Design review of the part shown in the three views and the two pictorial views. Dimensions are in mm from the part's minimum x, y and z. A direction names the side the tool comes from. Give positions to 0.01 mm unless a question says otherwise; leave off trailing zeros. Order: outer loops, then holes, each group sorted by start corner. A loop starts at its lowest first (then second) coordinate and runs counter-clockwise, first axis right, second up. Notation, with made-up numbers: (56, 77) -> (95, 77) arc R8 ccw to (95, 81) -> close; hole circle Ø2 at (-23.75, 53). An arc over 180 degrees is marked (long way). Use one line per item in the form item = value.
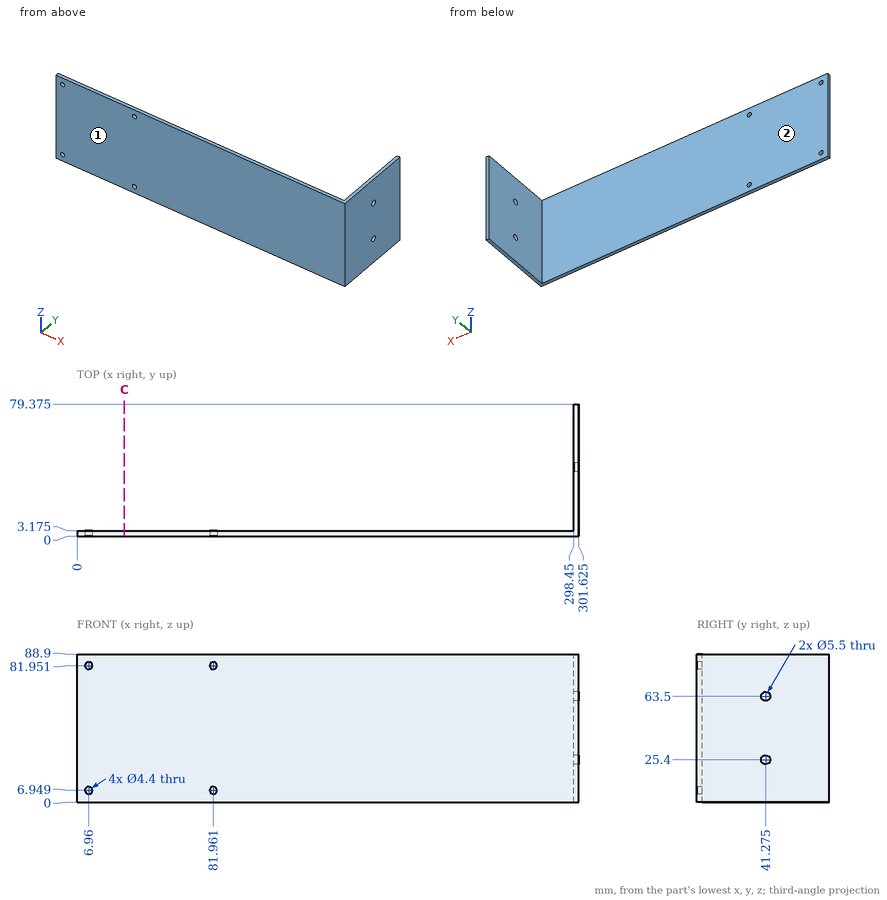
1. For L1, parallel to Y at x = 160, z = 70 (1 decimal), list the stretches that pass through material, from the lowest coordinate up.
Values:
L1 = 0 to 3.2
2. Add section C-C on x = 28.5. Give the boundary of the cut face in (y, z) (1 decimal).
Values:
outline = (0, 0) -> (3.2, 0) -> (3.2, 88.9) -> (0, 88.9) -> close
3. Tool access review of the marked faces 1 and 2: name each direction out of +Z, -Z, +X, -X, +Y, -Y from which nothing blocks a thin tool from reaching the whole face with its end or side.
Values:
face_1 = +Z, -Z, +X, -X, -Y
face_2 = +Z, -Z, -X, +Y
4. For pin 1 Ø5.5 at (x, z) = (81.96, 81.95) entering from +Y (3 decimals); pin 2 Ø1.5 at (y, z) = (60, 31.5) entering from -X, all flat-tipped, find the tip position at first contact; note any pin that passes through.
Values:
pin_1 = 3.175
pin_2 = 298.45
